from build123d import *

# Parameters (mm, degrees)
F5_DEPTH = 12.7


with BuildPart() as f3:
    # F0 (on Front) → F3 section 0
    with BuildSketch(Plane.XZ):
        Polygon((-19.05, 0), (0, 0), (19.05, 0), (19.05, 82.55), (0, 107.95), (-19.05, 82.55), align=None)
    # F2 (on offset) → F3 section 1
    with BuildSketch(Plane.XZ.offset(6.35)):
        Polygon((-12.7, 0), (0, 0), (12.7, 0), (12.7, 76.2), (0, 95.25), (-12.7, 76.2), align=None)
    loft()

    # F4 (on face) → F5 (join)
    with BuildSketch(Plane(origin=(0, 0, 0), x_dir=(1, 0, 0), z_dir=(0, 0, -1))):
        with BuildLine():
            Line((-1.0408426169, 0), (0, 0))
            Line((0, 0), (19.05, 0))
            add(Edge.make_bspline(
                [(19.05, 0), (12.7, 6.35)],
                knots=[0, 0, 1, 1], degree=1))
            Line((12.7, 6.35), (-12.7, 6.35))
            add(Edge.make_bspline(
                [(-19.05, 0), (-12.7, 6.35)],
                knots=[0, 0, 1, 1], degree=1))
            Line((-19.05, 0), (-1.0408426169, 0))
        make_face()
    extrude(amount=F5_DEPTH)


solid = f3.part
Verification items for the finished model (mm, model axes). Coordinates: 2 decimals unless noted, no trailing zeros. Order: outer loops, then holes, each group sorted by start corner. A loop starts at its lowest first (then second) coordinate and runs counter-clockwise, first axis right, second up. Notation, with made-up numbers: (43.25, 24) -> (84.25, 24) arc R13 cw to (84.25, 49) -> close; hole circle Ø2 at (15, -28.75). An arc over 180 degrees is marked (long way). Use CSV: the item, a comma, the result in double quotes. Start each with the question number.
Q1. Section check A-A, the plane z = 0. Record the cut outline in (x, y), and give its area (3 significant figures).
Q2. Depth check by flat-ended pin: P1, Ø1, axis at y = -1, z = 58.5, coming from the -X side; P2, Ø3, axis at x = 14.5, z = 38.5, coming from the +Y side; P3, Ø1, axis at y = -4.5, z = 35.5, coming from the +X side; P4, Ø2, axis at y = -1.5, z = 49, coming from the +X side. Enter the tip coordinate at first touch or a pass-through.
Q3. Thickness scan on line 1 along Z through (x, y) = (2, -2.5); line 2 along X through (y, z) = (-1.75, 73); line 3 along Y through (x, z) = (14.5, 8). Record the ranges inside material, lowest first.
Returned:
1,outline,"(-19.05, 0) -> (-12.7, -6.35) -> (12.7, -6.35) -> (19.05, 0) -> close"
1,area,"202 mm^2"
2,P1,"stops at x = -18.55"
2,P2,"stops at y = 0"
2,P3,"stops at x = 15.05"
2,P4,"stops at x = 18.55"
3,line 1,"z = -12.7 to 100.18"
3,line 2,"x = -17.3 to 17.3"
3,line 3,"y = -4.55 to 0"
